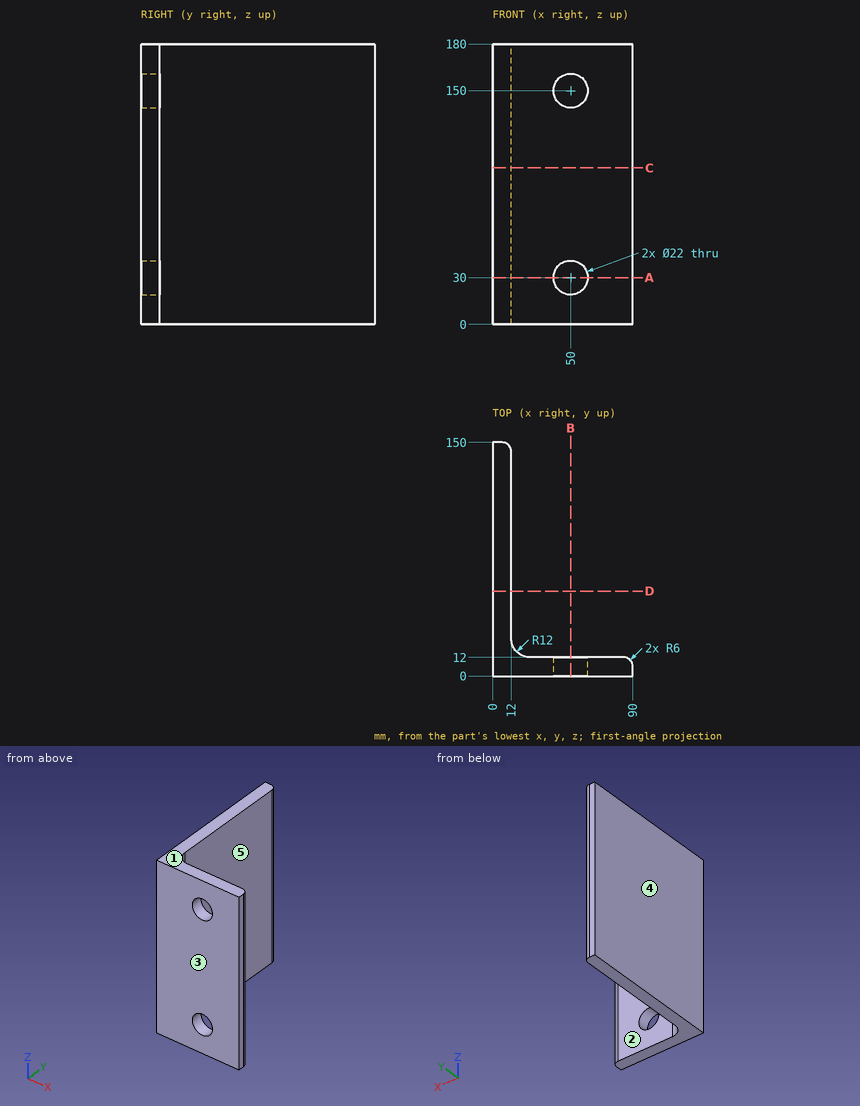
Study the drawing (mm; zero at the part's minimum x, y, z) and answer. A direction names the side the tool comes from. Give positions to 0.01 mm unless a question says otherwise; leave off trailing zeros. Write each loop counter-clockwise with the first axis right and the second up, starting at its lowest first coordinate (ties: lowest second). Pieces come first, ordered by that corner, then holes.
(1) The part is cut by section C-C on z = 100.5. Write down the section's boundary in (x, y).
Final values:
outline: (0, 0) - (90, 0) - (90, 6) arc R6 ccw to (84, 12) - (24, 12) arc R12 cw to (12, 24) - (12, 144) arc R6 ccw to (6, 150) - (0, 150) - close
(2) The mould has two halves that part along X. Classify the marked faces 3, 4 and 5: pulls with the +X half, pulls with the -X half, needs draft (parallel to the pull), parting line crosses it, or undercut.
Final values:
face 3: needs draft
face 4: pulls with the -X half
face 5: pulls with the +X half
(3) Flat-ended cylindrical pins translate along their axes: pin 1 Ø8 at (y, z) = (56, 106.5) entering from +X; pin 2 Ø1.5 at (x, z) = (10, 131) entering from +Y; pin 3 Ø20 at (x, z) = (50, 30) entering from +Y; pin 4 Ø12 at (x, z) = (64.5, 62) entering from +Y. Find the tip coordinate at first contact, or state that the pin passes through.
Final values:
pin 1: stops at x = 12
pin 2: stops at y = 149.04
pin 3: passes through
pin 4: stops at y = 12
(4) The part is cut by section D-D on y = 54.5. Write down the section's boundary in (x, z).
Final values:
outline: (0, 0) - (12, 0) - (12, 180) - (0, 180) - close
(5) Straight lines are drawn through the part: line 1 (Z direction, x = 50, y = 7); line 2 (Y direction, x = 73, z = 121.5). For each, find the intervals that lie inside material, in ascending order.
Final values:
line 1: z = 0 to 19, 41 to 139, 161 to 180
line 2: y = 0 to 12
(6) The part is cut by section B-B on x = 50. Write down the section's boundary in (y, z).
Final values:
outline: (0, 0) - (12, 0) - (12, 19) - (0, 19) - close; (0, 41) - (12, 41) - (12, 139) - (0, 139) - close; (0, 161) - (12, 161) - (12, 180) - (0, 180) - close
(7) Which of the six approach directions +Z, -Z, +X, -X, +Y, -Y give full straight-line access (tool end or side, diameter ignored) to the marked faces 1 and 2?
Final values:
face 1: +Z, +X, -X, +Y, -Y
face 2: +Z, -Z, +X, +Y
(8) The part is cut by section A-A on z = 30. Write down the section's boundary in (x, y).
Final values:
outline: (0, 0) - (39, 0) - (39, 12) - (24, 12) arc R12 cw to (12, 24) - (12, 144) arc R6 ccw to (6, 150) - (0, 150) - close; (61, 0) - (90, 0) - (90, 6) arc R6 ccw to (84, 12) - (61, 12) - close
